Here's how the part is built. I have some questions about the finished solid (model axes, mm). A direction names the side the tool comes from. Coordinates: 2 decimals unless noted, no trailing zeros. Write each loop counter-clockwise with the first axis right and the second up, starting at its lowest first coordinate (ties: lowest second). Pieces come first, ordered by that corner, then holes.
(1) Imagine slicing it at A-A, the plane x = -8. List the corners of the cut face in (y, z) for me, plus the area to 3 significant figures.
(2) Thinking about a two-plate mould opening in X: for faces 3 (the flat face through (-4, 0, -10)), 4 (the flat face through (-17.701, 1, -1)), 5 (the flat face through (13, 1, -3.206)), which applies, released by +X, released by -X, zero draft, split by the parting line, or undercut?
(3) Imagine slicing it at B-B, the plane z = -0.5. List the corners of the cut face in (x, y) for me.
(4) Please list where these lines run through material, in increasing order: probe 1 along X at (y, z) = (0.75, 3.75); probe 2 along X at (y, z) = (2.2, 1.5); probe 3 along Z at (x, y) = (-4, 1.25).
(5) For pin 1 Ø2 at (x, z) = (1.5, 7) entering from -Y, with a flat end and sliding along its axis, tell me the tip position at first contact or that it passes through.
(6) Imagine slicing it at C-C, the plane y = 0.7. List the corners of the cut face in (x, z) for me, plus the area to 3 significant figures.
(7) Which directions (+Z, -Z, +X, -X, +Y, -Y) give clear straight access to the entire face, cutting with the end or side of a thin tool? Please do faces 1 (the flat face through (0, 1, -14.517)), 2 (the flat face through (0, 1, -7.834)).
```python
from build123d import *

# Parameters (mm, degrees)
SKETCH2_W           = 35.12443
SKETCH2_H           = 27.47815276
SKETCH2_R           = 1.7
BOSS_EXTRUDE2_DEPTH = 2.5


with BuildPart() as part:
    # Sketch2 → Boss-Extrude2 (new body)
    with BuildSketch(Plane(origin=(0, 0, 0), x_dir=(1, 0, 0), z_dir=(0, 1, 0))):
        with Locations((-0.139276638, 0.7775026)):
            Rectangle(SKETCH2_W, SKETCH2_H)
        with Locations(Location((0.275439535, 11.02885898, 0), (0, 0, 270))):
            Circle(SKETCH2_R, mode=Mode.SUBTRACT)
        with Locations(Location((0, -9.47157378, 0), (0, 0, 270))):
            Circle(SKETCH2_R, mode=Mode.SUBTRACT)
        Polygon((-12.329001638, 7.83354898), (11.960588362, 7.83354898), (11.960588362, 3.2058826), (13.982538362, 3.2058826), (13.982538362, -1.6439074), (11.960588362, -1.6439074), (11.960588362, -6.27157378), (-12.329001638, -6.27157378), align=None, mode=Mode.SUBTRACT)
    extrude(amount=BOSS_EXTRUDE2_DEPTH)


solid = part.part
```
Recorded:
1. outline: (0, -14.52) - (2.5, -14.52) - (2.5, -7.83) - (0, -7.83) - close; (0, 6.27) - (2.5, 6.27) - (2.5, 12.96) - (0, 12.96) - close
1. area: 33.4 mm2
2. face 3: zero draft
2. face 4: released by -X
2. face 5: undercut
3. outline: (-17.7, 0) - (-12.33, 0) - (-12.33, 2.5) - (-17.7, 2.5) - close; (13.98, 0) - (17.42, 0) - (17.42, 2.5) - (13.98, 2.5) - close
4. probe 1: x = -17.7 to -12.33, 11.96 to 17.42
4. probe 2: x = -17.7 to -12.33, 13.98 to 17.42
4. probe 3: z = -14.52 to -7.83, 6.27 to 12.96
5. pin 1: stops at y = 0
6. outline: (-17.7, -14.52) - (17.42, -14.52) - (17.42, 12.96) - (-17.7, 12.96) - close; hole (-12.33, -7.83) - (11.96, -7.83) - (11.96, -3.21) - (13.98, -3.21) - (13.98, 1.64) - (11.96, 1.64) - (11.96, 6.27) - (-12.33, 6.27) - close; hole circle Ø3.4 at (0, 9.47); hole circle Ø3.4 at (0.28, -11.03)
6. area: 595 mm2
7. face 1: -Z, +X, -X, +Y, -Y
7. face 2: +Y, -Y
